For this review, take the finished solid that the model builds, in its own axes (mm). Round coordinates to 2 decimals unless told otherwise and drop trailing zeros. Write each loop counter-clockwise with the first axis right and the second up, starting at its lowest first coordinate (ties: lowest second). Pieces come first, ordered by that corner, then holes. Notation, with made-up numbers: (0.25, -4.75) -> (45.25, -4.75) arc R22 cw to (45.25, 1.25) -> close; hole circle Ø1 at (68, 60.25). An arc over 180 degrees is marked (long way). Answer in a Markdown table with one row per item. Add a question column.
Autodesk Inventor part; units mm, degrees
ref_plane "YZ Plane" through (0, 0, 0) normal (1, 0, 0) x (0, 1, 0)
ref_plane "XZ Plane" through (0, 0, 0) normal (0, 1, 0) x (-1, 0, 0)
ref_plane "XY Plane" through (0, 0, 0) normal (0, 0, 1) x (1, 0, 0)
sketch "Sketch1" plane through (0, 0, 0) normal (0, 0, 1) x (1, 0, 0)
  circle A0 centre (-6.35, 171.45) radius 2.1844
  circle A1 centre (6.35, 171.45) radius 2.1844
  circle A2 centre (23.8125, 120.65) radius 2.1844
  circle A3 centre (23.8125, 57.15) radius 2.1844
  circle A4 centre (-6.35, 57.15) radius 2.1844
  line L0 (-19.05, 52.07) -> (36.5125, 52.07)
  line L1 (36.5125, 52.07) -> (36.5125, 134.9375)
  line L2 (12.7, 184.15) -> (-19.05, 184.15)
  line L3 (-19.05, 184.15) -> (-19.05, 52.07)
  line L4 (12.7, 184.15) -> (12.7, 158.75)
  line L5 (12.7, 158.75) -> (36.5125, 134.9375)
  point P0 (0, 0)
  dimension "d0" = 12.7
  dimension "d2" = 12.7
  dimension "d3" = 5.08
  dimension "d4" = 12.7
  dimension "d15" = 25.4
  dimension "d16" = 31.75
  dimension "d17" = 135
extrude "Extrusion1" add sketch "Sketch1" along normal blind 2.54
fillet "Fillet1" radius 6.35 4 edges at (-19.05, 184.15, 1.27) (12.7, 184.15, 1.27) (12.7, 158.75, 1.27) (36.5125, 134.9375, 1.27)
chamfer "Chamfer1" distance 0.7937 angle 45 2 edges at (36.5125, 52.07, 1.27) (-19.05, 52.07, 1.27)
properties part number "funnelFront" material "white pla"
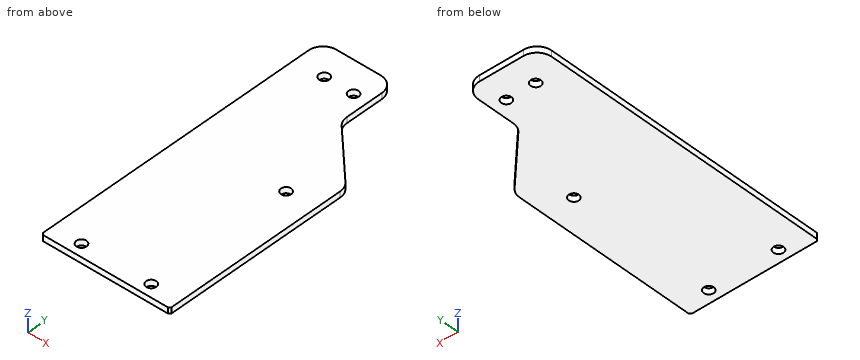
1. We need section C-C (x = -6.35). Write out the cut boundary in (y, z).
2. For L1, parallel to Y at x = -6.35, z = 1.75; L2, parallel to Y at x = 6.35, z = 1.9; L3, parallel to X at y = 166, z = 1.5, list the stretches that pass through material, from the lowest coordinate up. Write a range as [from, to].
3. We need section A-A (y = 57.15). Write out the cut boundary in (x, z).
4. We need section D-D (y = 176). Write out the cut boundary in (x, z), plus the area to 3 significant figures.
5. Clearance check with flat-ended pins moving along their axes: pin 1 Ø1.5 at (y, z) = (147.5, 1.5) entering from +X; pin 2 Ø2.5 at (x, y) = (23.81, 57.15) entering from -Z. State where each tip first meets the part, or that it passes through.
6. We need section B-B (y = 120.65). Write out the cut boundary in (x, z).
Response:
| question | item | result |
|---|---|---|
| 1 | outline | (52.07, 0) -> (54.97, 0) -> (54.97, 2.54) -> (52.07, 2.54) -> close; (59.33, 0) -> (169.27, 0) -> (169.27, 2.54) -> (59.33, 2.54) -> close; (173.63, 0) -> (184.15, 0) -> (184.15, 2.54) -> (173.63, 2.54) -> close |
| 2 | L1 | [52.07, 54.97], [59.33, 169.27], [173.63, 184.15] |
| 2 | L2 | [52.07, 169.27], [173.63, 184.15] |
| 2 | L3 | [-19.05, 12.7] |
| 3 | outline | (-19.05, 0) -> (-8.53, 0) -> (-8.53, 2.54) -> (-19.05, 2.54) -> close; (-4.17, 0) -> (21.63, 0) -> (21.63, 2.54) -> (-4.17, 2.54) -> close; (26, 0) -> (36.51, 0) -> (36.51, 2.54) -> (26, 2.54) -> close |
| 4 | outline | (-19.05, 0) -> (12.7, 0) -> (12.7, 2.54) -> (-19.05, 2.54) -> close |
| 4 | area | 80.6 mm2 |
| 5 | pin 1 | x = 24.7 |
| 5 | pin 2 | through |
| 6 | outline | (-19.05, 0) -> (21.63, 0) -> (21.63, 2.54) -> (-19.05, 2.54) -> close; (26, 0) -> (36.51, 0) -> (36.51, 2.54) -> (26, 2.54) -> close |
